```python
from build123d import *

# Parameters (mm, degrees)
F0_R     = 75
F0_W     = 7
F0_H     = 15
F1_DEPTH = 3
F2_DEPTH = 15
F3_R     = 2.5
F4_DEPTH = 99.4959988723
F5_R     = 8.5
F6_DEPTH = 2.5
F6_TAPER = 10


# Not quite as in the source:
# - a fillet or chamfer that OpenCascade refuses, or shapes differently, is made with other operations: its cross-section is extruded or revolved along the edge and cut away or added


with BuildPart() as f1:
    # F0 (on Top) → F1 (new body)
    with BuildSketch(Plane.XY):
        Circle(F0_R)
        with Locations((-20.9949988723, -60.5)):
            Rectangle(F0_W, F0_H, mode=Mode.SUBTRACT)
        with Locations((20.9949988723, -60.5)):
            Rectangle(F0_W, F0_H, mode=Mode.SUBTRACT)
        with Locations((-20.9949988723, -60.5)):
            Rectangle(F0_W, F0_H)
        with Locations((20.9949988723, -60.5)):
            Rectangle(F0_W, F0_H)
    extrude(amount=-F1_DEPTH)

    # F0 (on Top) → F2 (join)
    with BuildSketch(Plane.XY):
        with Locations((20.9949988723, -60.5)):
            Rectangle(F0_W, F0_H)
        with Locations((-20.9949988723, -60.5)):
            Rectangle(F0_W, F0_H)
    extrude(amount=F2_DEPTH)

    # F3 (on face) → F4 (cut, through all)
    with BuildSketch(Plane.YZ.offset(24.4949988723)):
        with BuildLine():
            ThreePointArc((-68, 7.5), (-65.8033008589, 12.8033008589), (-60.5, 15))
            Line((-60.5, 15), (-68, 15))
            Line((-68, 15), (-68, 7.5))
        make_face()
        with BuildLine():
            ThreePointArc((-60.5, 15), (-55.1966991411, 12.8033008589), (-53, 7.5))
            Line((-53, 7.5), (-53, 15))
            Line((-53, 15), (-60.5, 15))
        make_face()
        with Locations((-60.5, 10)):
            Circle(F3_R)
    extrude(amount=-F4_DEPTH, mode=Mode.SUBTRACT)

    # F5 (on face) → F6 (join)
    with BuildSketch(Plane.XY):
        with Locations((0, 63.5)):
            Circle(F5_R)
    extrude(amount=F6_DEPTH, taper=F6_TAPER)

    # F7: fillet of radius 5 on 1 edges, made by hand

    # F7_s1 → F7_t2 (revolve, cut)
    with BuildSketch(Plane.XZ.offset(-63.5)):
        with BuildLine():
            ThreePointArc((8.5, 0), (6.6698729811, 1.8301270189), (4.1698729811, 2.5))
            Line((4.1698729811, 2.5), (8.0591825482, 2.5))
            Line((8.0591825482, 2.5), (8.5, 0))
        make_face()
    revolve(axis=Axis((0, 63.5, 2.5), (0, 0, -1)), mode=Mode.SUBTRACT)


solid = f1.part
```
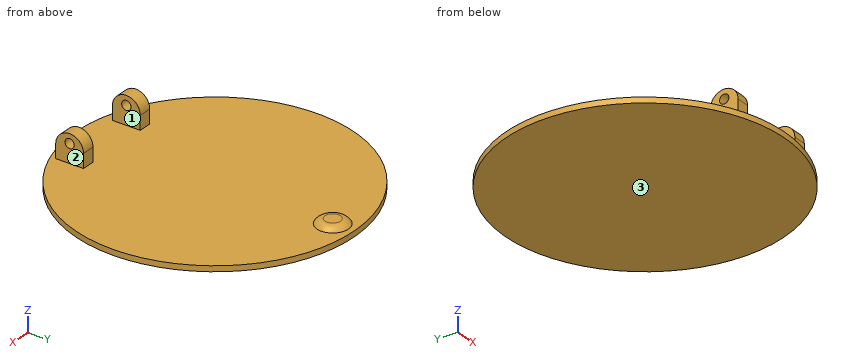
Model file for the job. Use its own axes, mm. Face numbers are marked on the shaded views. A direction names the side the tool comes from. Coordinates: 2 decimals unless noted, no trailing zeros. Write each loop counter-clockwise with the first axis right and the second up, starting at its lowest first coordinate (ties: lowest second). Pieces come first, ordered by that corner, then holes. Notation, with made-up numbers: (-38, 34) - (-22, 34) arc R34 ccw to (-22, 65) - close; hole circle Ø6 at (82.25, 60.25). An arc over 180 degrees is marked (long way). One line per question, with ' | ' between items. Start each with the question number.
Q1. Cut at A-A, the plane z = 4.5. List the corners of the cut face in (x, y) (3 decimals), then the cut area to 3 significant figures.
Q2. Cut at D-D, the plane x = -33.5. List the corners of the cut face in (y, z), then the cut area to 3 significant figures.
Q3. 3-axis set-ups, long thin cutter, end or side, ignore diameter. For the marked faces 1, 2 and 3: which of +Z, -Z, +X, -X, +Y, -Y reach the whole face in a straight line?
Q4. Drill centre lines: line 1 (X direction, y = -61.5, z = 3.75) (3 decimals); line 2 (Z direction, x = 66, y = 16.5); line 3 (Y direction, x = -24, z = 9). Where is each one in solid material? Low to high. Write a range as [from, to].
Q5. Pin check, flat tips, straight feed: pin 1 (7.5 mm diameter, centred on y = -60.5, z = 6, fed in from -X) (3 decimals); pin 2 (8 mm diameter, centred on x = 52, z = 0.5, fed in from -Y); pin 3 (2 mm diameter, centred on x = -21.5, z = 2.5, fed in from +Y); pin 4 (12 mm diameter, centred on x = 58.5, y = 57.5, fed in from -Z). Stop position of each tip, or through.
Q6. Cut at C-C, the plane y = 0. List the corners of the cut face in (x, z).
Q7. Cut at B-B, the plane y = -60.5. List the corners of the cut face in (x, z) (1 decimal).
Answer below:
1) outline: (-24.495, -68) - (-17.495, -68) - (-17.495, -53) - (-24.495, -53) - close; (17.495, -68) - (24.495, -68) - (24.495, -53) - (17.495, -53) - close | area: 210 mm^2
2) outline: (-67.1, -3) - (67.1, -3) - (67.1, 0) - (-67.1, 0) - close | area: 403 mm^2
3) face 1: +Z, +Y, -Y | face 2: +Z, +X, +Y, -Y | face 3: -Z, +X, -X, +Y, -Y
4) line 1: [-24.495, -17.495], [17.495, 24.495] | line 2: [-3, 0] | line 3: [-67.85, -62.79], [-58.21, -53.15]
5) pin 1: x = -24.495 | pin 2: y = -57.6 | pin 3: y = -53 | pin 4: through
6) outline: (-75, -3) - (75, -3) - (75, 0) - (-75, 0) - close
7) outline: (-44.3, -3) - (44.3, -3) - (44.3, 0) - (24.5, 0) - (24.5, 7.5) - (17.5, 7.5) - (17.5, 0) - (-17.5, 0) - (-17.5, 7.5) - (-24.5, 7.5) - (-24.5, 0) - (-44.3, 0) - close; (-24.5, 12.5) - (-17.5, 12.5) - (-17.5, 15) - (-24.5, 15) - close; (17.5, 12.5) - (24.5, 12.5) - (24.5, 15) - (17.5, 15) - close
